The listing builds one solid part. Answer for the finished solid, in the listing's coordinates (mm). Coordinates: 2 decimals unless noted, no trailing zeros. Loops run counter-clockwise (first coordinate to the right, second up) from the corner with the lowest first, then second, coordinate; pieces in that order, holes last. Notation, with made-up numbers: (16.25, 24) - (50.25, 24) arc R19 ccw to (50.25, 45) - close; hole circle Ø7 at (63.25, 50.25). An arc over 180 degrees is marked (long way). Use one line per item in the form item = value. Start each with the question number.
```python
from build123d import *

# Parameters (mm, degrees)
SKETCH_1_W         = 24
SKETCH_1_H         = 16
EXTRUDE_1_DEPTH    = 27
SKETCH1_R          = 1.5
CUT_EXTRUDE1_DEPTH = 34.600595233


with BuildPart() as part:
    # 草图1 → 凸台-拉伸1 (new, symmetric)
    with BuildSketch(Plane.XY):
        Rectangle(SKETCH_1_W, SKETCH_1_H)
    extrude(amount=EXTRUDE_1_DEPTH, both=True)

    # Sketch1 → Cut-Extrude1 (cut, through all)
    with BuildSketch(Plane(origin=(0, 8, 0), x_dir=(1, 0, 0), z_dir=(0, 1, 0))):
        with Locations(Location((-9.5, 17, 0), (0, 0, 180))):
            Circle(SKETCH1_R)
        with Locations((9.5, 17)):
            Circle(SKETCH1_R)
        with Locations(Location((9.5, -17, 0), (0, 0, 180))):
            Circle(SKETCH1_R)
        with Locations((-9.5, -17)):
            Circle(SKETCH1_R)
    extrude(amount=-CUT_EXTRUDE1_DEPTH, mode=Mode.SUBTRACT)


solid = part.part
```
(1) A cutting plane is placed at A-A (z = -17). Determine the outline of the cut face in (x, y).
(2) This flat-tipped pin is pushed along its axis until it touches: pin 1 Ø2.5 at (x, z) = (-9.5, -17) entering from -Y. Where does it stop, or does it pass through?
(3) Determine the mould class of faces 1 (the face through (12, 0, 0)), 2 (the face through (0, 0, 27)), 3 (the face through (-8.39, 0.11, -15.99)) for opening direction Z: +Z half, -Z half, draft (parallel to the pull), parting line (faces both ways), or undercut.
(4) A cutting plane is placed at C-C (x = -9.5). Determine the outline of the cut face in (y, z).
(5) Find the intervals of material crossed by probe 1 along Z at (x, y) = (-9.5, 1.5), in increasing order. Write a range as from..to.
(6) A cutting plane is placed at B-B (y = 0). Determine the outline of the cut face in (x, z), then the cut area to 3 significant figures.
Evaluation:
q1.outline = (-12, -8) - (-11, -8) - (-11, 8) - (-12, 8) - close; (-8, -8) - (8, -8) - (8, 8) - (-8, 8) - close; (11, -8) - (12, -8) - (12, 8) - (11, 8) - close
q2.pin_1 = through
q3.face_1 = draft
q3.face_2 = +Z half
q3.face_3 = undercut
q4.outline = (-8, -27) - (8, -27) - (8, -18.5) - (-8, -18.5) - close; (-8, -15.5) - (8, -15.5) - (8, 15.5) - (-8, 15.5) - close; (-8, 18.5) - (8, 18.5) - (8, 27) - (-8, 27) - close
q5.probe_1 = -27..-18.5, -15.5..15.5, 18.5..27
q6.outline = (-12, -27) - (12, -27) - (12, 27) - (-12, 27) - close; hole circle Ø3 at (-9.5, -17); hole circle Ø3 at (-9.5, 17); hole circle Ø3 at (9.5, -17); hole circle Ø3 at (9.5, 17)
q6.area = 1,270 mm^2
